Source: CAD feature listing. Evaluate the final solid. Frame: model axes, mm. A direction names the side the tool comes from. Round coordinates to 2 decimals unless told otherwise and drop trailing zeros. Order: outer loops, then holes, each group sorted by start corner. A loop starts at its lowest first (then second) coordinate and runs counter-clockwise, first axis right, second up. Notation, with made-up numbers: (9.25, -23.5) - (41.25, -23.5) arc R28 cw to (41.25, 7.5) - close; hole circle Ø10 at (-39, -16.5). An arc over 180 degrees is marked (long way). Use one line per item in the form item = value. Start each with the question number.
Q1. Pin query (flat end, axial travel): pin 1 Ø2 at (y, z) = (3, 3.5) entering from +X; pin 2 Ø4 at (x, y) = (0.5, -2.5) entering from -Z; pin 3 Ø8 at (x, z) = (8.5, 11) entering from +Y. Return the tip coordinate at first contact, or that it passes through.
Q2. Set-up query: faces 1 (the cylindrical face through (-2.248, 0.099, 9.633)), 2 (the flat face through (6.928, 0, -3)). Return all of +Z, -Z, +X, -X, +Y, -Y with unobstructed straight access to the full face (end or side cutting, diameter ignored); none if empty.
Q3. Ray query, line 1 (Y direction, x = 0, z = 4.5); line 2 (Z direction, x = 12, y = 0); line 3 (Z direction, x = 6, y = 0). Return the intervals inside material, ascending. Write a range as [from, to].
Q4. Cut plane A-A, the plane y = 0. Return the cut outline in (x, z), and give its area (3 significant figures).
Q5. Cut plane D-D, the plane y = 12. Return the cut outline in (x, z), and give its area (3 significant figures).
Q6. Cut plane B-B, the plane x = -5. Return the cut outline in (y, z), and give its area (3 significant figures).
Q7. Cut plane C-C, the plane z = 12. Return the cut outline in (x, y).
Q8. Draft query along Z for faces 3 (the flat face through (0, -3, 19)), 4 (the flat face through (2, -2, 0)), 5 (the flat face through (-3.513, -5.972, -2.535)), 6 (the cylindrical face through (8.29, -0.18, 13.61)). Return one class per face: released by +Z, released by -Z, zero draft, split by the parting line, or undercut.
Autodesk Inventor part; units mm, degrees
ref_plane "YZ Plane" through (0, 0, 0) normal (1, 0, 0) x (0, 1, 0)
ref_plane "XZ Plane" through (0, 0, 0) normal (0, 1, 0) x (-1, 0, 0)
ref_plane "XY Plane" through (0, 0, 0) normal (0, 0, 1) x (1, 0, 0)
sketch "Sketch1" plane through (0, 0, 0) normal (0, 0, 1) x (1, 0, 0)
  circle A0 centre (0, 0) radius 15
  dimension "d0" = 30
extrude "Extrusion1" add sketch "Sketch1" along normal blind 19
sketch "Sketch2" plane through (0, 0, 19) normal (0, 0, 1) x (1, 0, 0)
  circle A0 centre (0, 0) radius 2.25
  dimension "d3" = 4.5
extrude "Extrusion2" cut sketch "Sketch2" against normal blind 19
sketch "Sketch3" plane through (0, 0, 0) normal (0, 0, -1) x (-1, 0, 0)
  circle A0 centre (0, 0) radius 15
extrude "Extrusion3" add sketch "Sketch3" along normal blind 5
sketch "Sketch6" plane through (0, 0, -5) normal (0, 0, -1) x (-1, 0, 0)
  line L0 (0, -8) -> (-6.9282, -4)
  line L1 (-6.9282, -4) -> (-6.9282, 4)
  line L2 (-6.9282, 4) -> (0, 8)
  line L3 (0, 8) -> (6.9282, 4)
  line L4 (6.9282, 4) -> (6.9282, -4)
  line L5 (6.9282, -4) -> (0, -8)
  point P0 (0, 0)
  point P1 (0, 0)
  dimension "d15" = 16
extrude "Extrusion6" cut sketch "Sketch6" against normal blind 5
sketch "Sketch7" plane through (0, 0, 0) normal (1, 0, 0) x (0, 1, 0)
  circle A0 centre (0, 15) radius 1.4
  line L0 (15, 19) -> (-15, 19)
  point P0 (0, 0)
  dimension "d18" = 2.8
  dimension "d22" = 4
extrude "Extrusion7" cut sketch "Sketch7" along normal through all
properties part number "AA009" material "ABS Plastic"
Completed:
q1.pin_1 = 14.87
q1.pin_2 = 0
q1.pin_3 = 14.31
q2.face_1 = +Z, -Z
q2.face_2 = -Z
q3.line_1 = [-15, -2.25], [2.25, 15]
q3.line_2 = [-5, 13.6], [16.4, 19]
q3.line_3 = [0, 13.6], [16.4, 19]
q4.outline = (-15, -5) - (-6.93, -5) - (-6.93, 0) - (-2.25, 0) - (-2.25, 19) - (-15, 19) - close; (2.25, 0) - (6.93, 0) - (6.93, -5) - (15, -5) - (15, 13.6) - (2.25, 13.6) - close; (2.25, 16.4) - (15, 16.4) - (15, 19) - (2.25, 19) - close
q4.area = 530 mm2
q5.outline = (-9, -5) - (9, -5) - (9, 19) - (-9, 19) - close
q5.area = 432 mm2
q6.outline = (-14.14, -5) - (-5.11, -5) - (-5.11, 0) - (5.11, 0) - (5.11, -5) - (14.14, -5) - (14.14, 19) - (-14.14, 19) - close
q6.area = 628 mm2
q7.outline = circle Ø30 at (0, 0); hole circle Ø4.5 at (0, 0)
q8.face_3 = released by +Z
q8.face_4 = released by -Z
q8.face_5 = zero draft
q8.face_6 = undercut
